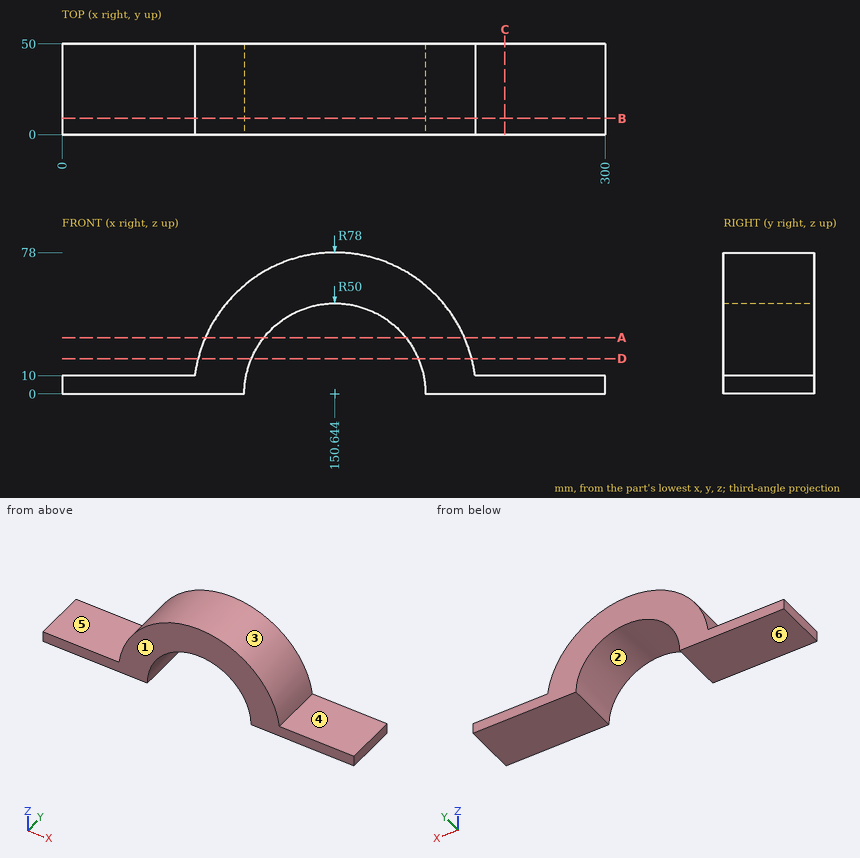
Here's the drawing with two shaded views (mm, measured from the low corner). I have some questions. A direction names the side the tool comes from. Round coordinates to 2 decimals unless told otherwise and drop trailing zeros. Order: outer loops, then holes, each group sorted by start corner. A loop starts at its lowest first (then second) coordinate and runs counter-clockwise, first axis right, second up. Notation, with made-up numbers: (19, 48) -> (42, 48) arc R21 cw to (42, 55) -> close; hole circle Ø9 at (-24, 86). An arc over 180 degrees is marked (long way). Use a Markdown table: item, result. Add a question column.
(1) I need wall thicknesses on line 1 along Z through (x, y) = (283, 31.5); line 2 along X through (y, z) = (12.5, 32) (1 decimal); line 3 along X through (y, z) = (43, 8). Which ranges of each line are inside material? Lowest first, please.
(2) Suppose I cut it at C-C, the plane x = 244.5. Please give me the cut outline in (y, z), and give its area (3 significant figures).
(3) For the marked faces 4, 5 and 6, which set-ups out of +Z, -Z, +X, -X, +Y, -Y let a thin tool reach every point of the face, with its end or its side?
(4) Suppose I cut it at D-D, the plane z = 19.5. Please give me the cut outline in (x, y) (1 decimal).
(5) For pin 1 Ø5 at (x, y) = (218, 40.5) entering from +Z; pin 2 Ø8 at (x, y) = (153.5, 12.5) entering from +Z; pin 3 Ø5 at (x, y) = (133, 8.5) entering from +Z, each with a flat end and sliding along its axis, tell me the tip position at first contact or that it passes through.
(6) Suppose I cut it at A-A, the plane z = 31. Please give me the cut outline in (x, y).
(7) Suppose I cut it at B-B, the plane y = 9. Please give me the cut outline in (x, z), and give its area (3 significant figures).
(8) If we mould it in two halves opening along X, with no side actions, what happens to the marked faces 1, 2 and 3? For each: released by +X, released by -X, zero draft, split by the parting line, or undercut.
Verdict:
| question | item | result |
|---|---|---|
| 1 | line 1 | 0 to 10 |
| 1 | line 2 | 79.5 to 112.2, 189.1 to 221.8 |
| 1 | line 3 | 0 to 101.29, 200 to 300 |
| 2 | outline | (0, 0) -> (50, 0) -> (50, 10) -> (0, 10) -> close |
| 2 | area | 500 mm2 |
| 3 | face 4 | +Z, +X, +Y, -Y |
| 3 | face 5 | +Z, -X, +Y, -Y |
| 3 | face 6 | -Z, +X, -X, +Y, -Y |
| 4 | outline | (75.1, 0) -> (104.6, 0) -> (104.6, 50) -> (75.1, 50) -> close; (196.7, 0) -> (226.2, 0) -> (226.2, 50) -> (196.7, 50) -> close |
| 5 | pin 1 | z = 43.33 |
| 5 | pin 2 | z = 78 |
| 5 | pin 3 | z = 76.52 |
| 6 | outline | (79.07, 0) -> (111.41, 0) -> (111.41, 50) -> (79.07, 50) -> close; (189.87, 0) -> (222.22, 0) -> (222.22, 50) -> (189.87, 50) -> close |
| 7 | outline | (0, 0) -> (100.64, 0) arc R50 cw to (200.64, 0) -> (300, 0) -> (300, 10) -> (228, 10) arc R78 ccw to (73.29, 10) -> (0, 10) -> close |
| 7 | area | 7,070 mm2 |
| 8 | face 1 | zero draft |
| 8 | face 2 | undercut |
| 8 | face 3 | split by the parting line |
